Drawing for the job (mm, zero at the part's lowest x, y, z). A direction names the side the tool comes from. Give positions to 0.01 mm unless a question says otherwise; leave off trailing zeros. Loops run counter-clockwise (first coordinate to the right, second up) from the corner with the lowest first, then second, coordinate; pieces in that order, holes last.
1) Band-saw the part on A-A on z = 5. State how many separate pieces and enclosed holes the cut face has, then the cut area to 3 significant figures.
2) Two-plate mould, pull along Y, no slides. Class the marked faces 1, 2, 3 and 4: +Y half, -Y half, draft (parallel to the pull), parting line (faces both ways), or undercut.
3) Flat gauge pins, fed straight in: P1, Ø1.5, axis at x = 23, y = 5.5, coming from the -Z side; P2, Ø3, axis at y = 15.5, z = 7, coming from the +X side (1 decimal); P3, Ø0.6, axis at y = 19, z = 4.5, coming from the +X side (1 decimal); P4, Ø5, axis at y = 12.5, z = 5.5, coming from the +X side. Where does each tip first touch, or does it go through?
4) Band-saw the part on D-D on x = 35. List the corners of the cut face in (y, z).
5) 3-axis set-ups, long thin cutter, end or side, ignore diameter. For the marked faces 5, 6 and 7: which of +Z, -Z, +X, -X, +Y, -Y reach the whole face in a straight line?
6) Band-saw the part on C-C on x = 15. List the corners of the cut face in (y, z).
7) Band-saw the part on B-B on y = 18.5. List the corners of the cut face in (x, z) (1 decimal).
8) Wall check: line 1 (X direction, y = 1.5, z = 5); line 2 (X direction, y = 18.95, z = 5) (1 decimal); line 3 (Y direction, x = 30, z = 5.5). Give the ranges that are in metal, low to high.
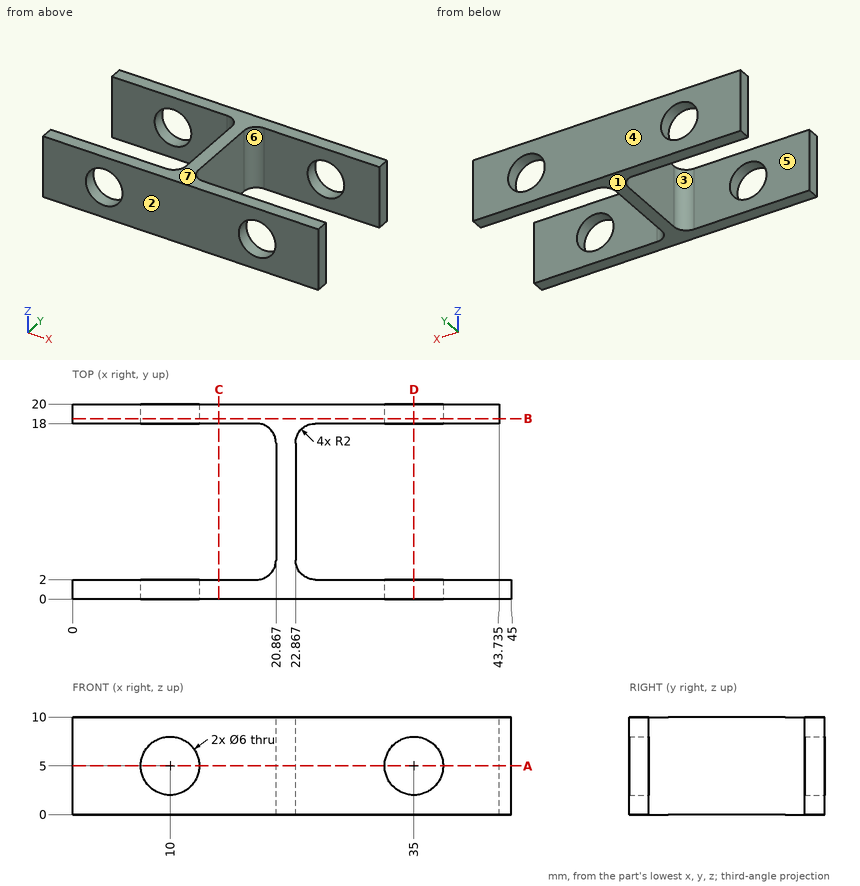
Findings below:
1. separate pieces: 5
1. enclosed holes: 0
1. area: 165 mm2
2. face 1: draft
2. face 2: -Y half
2. face 3: undercut
2. face 4: +Y half
3. P1: stops at z = 0
3. P2: stops at x = 23.1
3. P3: stops at x = 43.7
3. P4: stops at x = 22.87
4. outline: (0, 0) - (2, 0) - (2, 2) - (0, 2) - close; (0, 8) - (2, 8) - (2, 10) - (0, 10) - close; (18, 0) - (20, 0) - (20, 2) - (18, 2) - close; (18, 8) - (20, 8) - (20, 10) - (18, 10) - close
5. face 5: +Z, -Z, -X
5. face 6: +Z, -Z, +X
5. face 7: +Z, +X, -X, +Y, -Y
6. outline: (0, 0) - (2, 0) - (2, 10) - (0, 10) - close; (18, 0) - (20, 0) - (20, 10) - (18, 10) - close
7. outline: (0, 0) - (43.7, 0) - (43.7, 10) - (0, 10) - close; hole circle Ø6 at (10, 5); hole circle Ø6 at (35, 5)
8. line 1: x = 0 to 7, 13 to 32, 38 to 45
8. line 2: x = 0 to 7, 13 to 32, 38 to 43.7
8. line 3: y = 0 to 2, 18 to 20
